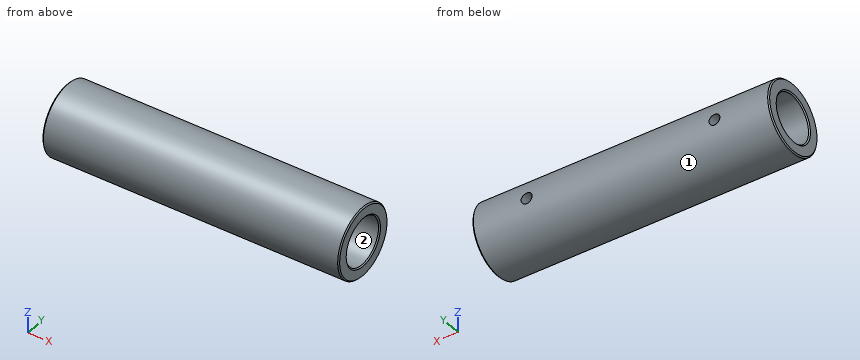
```python
from build123d import *

# Parameters (mm, degrees)
SKETCH_1_R              = 45
SKETCH_1_R_2            = 30
EXTRUDE_1_DEPTH         = 379
CHAMFER_1_SIZE          = 1.5
HOLE_WIZARD_M16_2_D     = 14
HOLE_WIZARD_M16_2_DEPTH = 42
HOLE_WIZARD_M16_2_TIP   = 4.206024333


with BuildPart() as part:
    # 草图1 → 凸台-拉伸1 (new body)
    with BuildSketch(Plane(origin=(0, 0, 0), x_dir=(0, 0, -1), z_dir=(1, 0, 0))):
        Circle(SKETCH_1_R)
        Circle(SKETCH_1_R_2, mode=Mode.SUBTRACT)
    extrude(amount=EXTRUDE_1_DEPTH)

    # 倒角1
    chamfer_1_edges = [part.edges().sort_by_distance(p)[0] for p in [
        (0, 0, 45),
        (379, 0, 45),
        (0, 0, 30),
        (379, 0, 30),
    ]]
    chamfer(chamfer_1_edges, length=CHAMFER_1_SIZE)

    # M16 螺纹孔2
    with Locations(Plane(origin=(0, 45, 0), x_dir=(1, 0, 0), z_dir=(0, 1, 0))):
        with Locations((69.5, 0), (309.5, 0)):
            Hole(HOLE_WIZARD_M16_2_D / 2, depth=HOLE_WIZARD_M16_2_DEPTH)
            with Locations((0, 0, -(HOLE_WIZARD_M16_2_DEPTH + HOLE_WIZARD_M16_2_TIP / 2))):  # 118° drill point
                Cone(0, HOLE_WIZARD_M16_2_D / 2, HOLE_WIZARD_M16_2_TIP, mode=Mode.SUBTRACT)


solid = part.part
```
For this review, take the finished solid that the model builds, in its own axes (mm). Face numbers are marked on the shaded views. Round coordinates to 2 decimals unless told otherwise and drop trailing zeros. Write each loop counter-clockwise with the first axis right and the second up, starting at its lowest first coordinate (ties: lowest second). Pieces come first, ordered by that corner, then holes. Notation, with made-up numbers: (4, 29.25) -> (57, 29.25) arc R31 ccw to (57, 66.25) -> close; hole circle Ø9 at (-3, -18.5). An arc over 180 degrees is marked (long way). Use one line per item in the form item = value.
1) Mouldability with a two-part tool opening along Z and no side actions: class the marked faces 1 and 2 as +Z half, -Z half, draft (parallel to the pull), parting line (faces both ways), or undercut.
Found:
face_1 = parting line
face_2 = undercut
2) Take a section at B-B, the plane x = 346.5. Write out the cut boundary in (y, z), and give its area (3 significant figures).
Found:
outline = circle Ø90 at (0, 0); hole circle Ø60 at (0, 0)
area = 3,530 mm2
3) Clearance check with flat-ended pins moving along their axes: pin 1 (3 mm diameter, centred on x = 55, z = 5.5, fed in from -Y); pin 2 (4 mm diameter, centred on x = 164, y = 18, fed in from -Z); pin 3 (8 mm diameter, centred on x = 92.5, y = 13.5, fed in from -Z). State where each tip first meets the part, or that it passes through.
Found:
pin_1 = -44.82
pin_2 = -42.06
pin_3 = -43.99
4) Take a section at A-A, the plane y = 0. Write out the cut boundary in (x, z), and give its area (3 significant figures).
Found:
outline = (0, -43.5) -> (1.5, -45) -> (377.5, -45) -> (379, -43.5) -> (379, -31.5) -> (377.5, -30) -> (1.5, -30) -> (0, -31.5) -> close; (0, 31.5) -> (1.5, 30) -> (377.5, 30) -> (379, 31.5) -> (379, 43.5) -> (377.5, 45) -> (1.5, 45) -> (0, 43.5) -> close
area = 11,400 mm2
5) Take a section at C-C, the plane y = 39.5. Count the separate pieces of the cut face and the enclosed holes in it, and give its area (3 significant figures).
Found:
separate_pieces = 1
enclosed_holes = 2
area = 16,000 mm2
6) To check wall thickness, follow L1, parallel to Y at x = 89, z = 0; L2, parallel to Z at x = 69.5, y = 38.5; L3, parallel to Y at x = 74.5, z = 27. State the ranges of each line that lie inside material, in increasing order. Write a range as from..to.
Found:
L1 = -45..-30, 30..45
L2 = -23.3..-7, 7..23.3
L3 = -36..-13.08, 13.08..36
